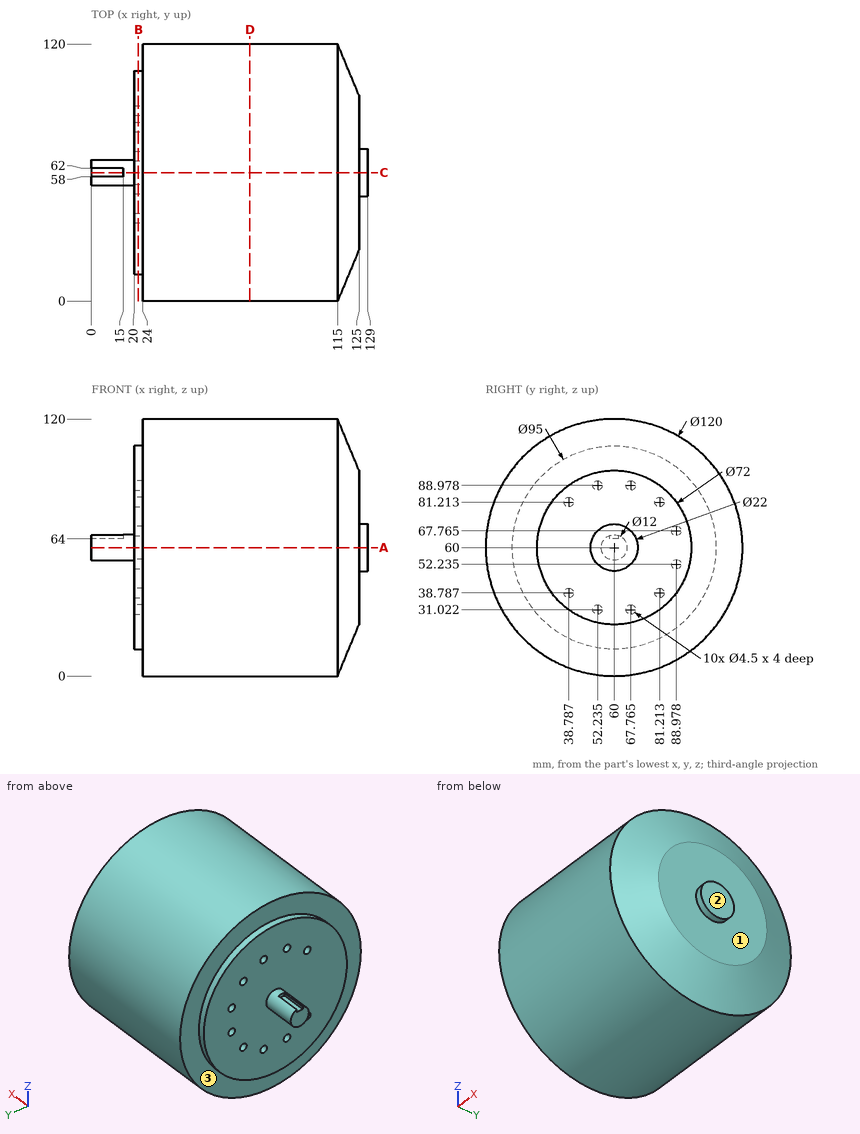
Study the drawing (mm; zero at the part's minimum x, y, z) and answer. A direction names the side the tool comes from. Give positions to 0.01 mm unless a question says otherwise; leave off trailing zeros. Write each loop counter-clockwise with the first axis right and the second up, starting at its lowest first coordinate (ties: lowest second). Pieces come first, ordered by that corner, then holes. Notation, with made-up numbers: (77, 57.5) -> (104, 57.5) arc R24 ccw to (104, 94.5) -> close; hole circle Ø2 at (-0.75, -9.75). An arc over 180 degrees is marked (long way). Write item = value, one per line. Start each with the question number.
1) The part is cut by section A-A, the plane z = 60. Determine the outline of the cut face in (x, y).
2) Which of the six approach directions +Z, -Z, +X, -X, +Y, -Y give full straight-line access (tool end or side, diameter ignored) to the marked faces 1, 2 and 3?
3) The part is cut by section D-D, the plane x = 74. Determine the outline of the cut face in (y, z), and give its area (3 significant figures).
4) Each of these flat-tipped pins is pushed along its axis until it touches: pin 1 (1.8 mm diameter, centred on x = 5.5, z = 65, fed in from -Y); pin 2 (4 mm diameter, centred on y = 67.76, z = 31.02, fed in from +X); pin 3 (8 mm diameter, centred on x = 94.5, z = 104, fed in from +Y). Where does it stop, or does it pass through?
5) The part is cut by section B-B, the plane x = 22. Count the separate pieces of the cut face and the enclosed holes in it, and give its area (3 significant figures).
6) Straight lines are drawn through the part: line 1 along X through (y, z) = (57, 47); line 2 along X through (y, z) = (44.5, 14.5); line 3 along Y through (x, z) = (32.5, 16.5) (1 decimal). For each, find the intervals that lie inside material, in ascending order.
7) The part is cut by section C-C, the plane y = 60. Determine the outline of the cut face in (x, z).
Solutions:
q1.outline = (0, 54) -> (20, 54) -> (20, 12.5) -> (24, 12.5) -> (24, 0) -> (115, 0) -> (125, 24) -> (125, 49) -> (129, 49) -> (129, 71) -> (125, 71) -> (125, 96) -> (115, 120) -> (24, 120) -> (24, 107.5) -> (20, 107.5) -> (20, 66) -> (0, 66) -> close
q2.face_1 = +X
q2.face_2 = +Z, -Z, +X, +Y, -Y
q2.face_3 = -X
q3.outline = circle Ø120 at (60, 60)
q3.area = 11,300 mm²
q4.pin_1 = 55.62
q4.pin_2 = 125
q4.pin_3 = 104.72
q5.separate_pieces = 1
q5.enclosed_holes = 10
q5.area = 6,930 mm²
q6.line_1 = 20 to 125
q6.line_2 = 24 to 119.97
q6.line_3 = 18.7 to 101.3
q7.outline = (0, 54) -> (20, 54) -> (20, 12.5) -> (24, 12.5) -> (24, 0) -> (115, 0) -> (125, 24) -> (125, 49) -> (129, 49) -> (129, 71) -> (125, 71) -> (125, 96) -> (115, 120) -> (24, 120) -> (24, 107.5) -> (20, 107.5) -> (20, 66) -> (15, 66) -> (15, 64) -> (0, 64) -> close
